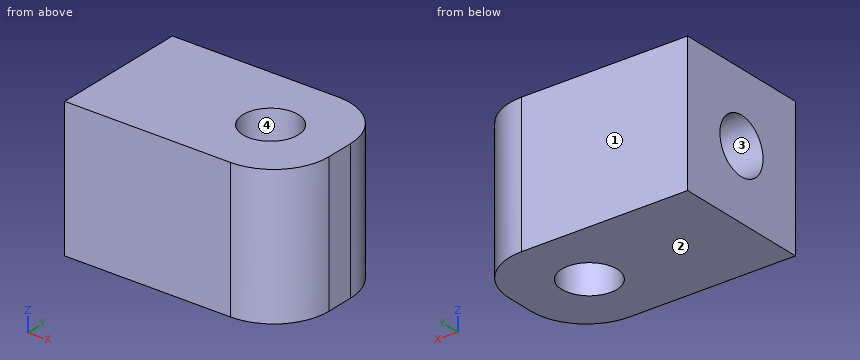
from build123d import *

# Parameters (mm, degrees)
SKETCH1_W           = 8
SKETCH1_H           = 5
BOSS_EXTRUDE1_DEPTH = 5
SKETCH2_R           = 1
CUT_EXTRUDE1_DEPTH  = 4
SKETCH3_R           = 1
CUT_EXTRUDE4_DEPTH  = 5
FILLET1_R           = 2


with BuildPart() as part:
    # Sketch1 → Boss-Extrude1 (new body)
    with BuildSketch(Plane.XY):
        with Locations((4, 2.5)):
            Rectangle(SKETCH1_W, SKETCH1_H)
    extrude(amount=BOSS_EXTRUDE1_DEPTH)

    # Sketch2 → Cut-Extrude1 (cut)
    with BuildSketch(Plane.ZY):
        with Locations((2.5, 2.5)):
            Circle(SKETCH2_R)
    extrude(amount=-CUT_EXTRUDE1_DEPTH, mode=Mode.SUBTRACT)

    # Sketch3 → Cut-Extrude4 (cut)
    with BuildSketch(Plane.XY.offset(5)):
        with Locations((5.5, 2.5)):
            Circle(SKETCH3_R)
    extrude(amount=-CUT_EXTRUDE4_DEPTH, mode=Mode.SUBTRACT)

    # Fillet1
    fillet1_edges = [part.edges().sort_by_distance(p)[0] for p in [
        (8, 5, 2.5),
        (8, 0, 2.5),
    ]]
    fillet(fillet1_edges, radius=FILLET1_R)


solid = part.part
Check sheet for the modelled part. Datum: model origin and axes. Units: mm. Face numbers are marked on the shaded views. Give positions to 0.01 mm unless a question says otherwise; leave off trailing zeros. Order: outer loops, then holes, each group sorted by start corner. A loop starts at its lowest first (then second) coordinate and runs counter-clockwise, first axis right, second up. Notation, with made-up numbers: (69.5, 21.5) - (122.5, 21.5) arc R18 ccw to (122.5, 41.5) - close; hole circle Ø1 at (-4, -19.5). An arc over 180 degrees is marked (long way). Answer as CSV lines item,"result".
1. Section check D-D (z = 3.75). Record the boundary of the cut face in (x, y).
Result sheet:
outline,"(0, 0) - (6, 0) arc R2 ccw to (8, 2) - (8, 3) arc R2 ccw to (6, 5) - (0, 5) - close; hole circle Ø2 at (5.5, 2.5)"
2. Section check A-A (x = 5.5). Record the boundary of the cut face in (y, z), then the cut area to 3 significant figures.
Result sheet:
outline,"(0, 0) - (1.5, 0) - (1.5, 5) - (0, 5) - close; (3.5, 0) - (5, 0) - (5, 5) - (3.5, 5) - close"
area,"15.0 mm²"
3. Mould release check, pull along Y, two halves, no side actions. Record for the marked faces 1, 2, 3 and 4: released by +Y, released by -Y, zero draft, split by the parting line, or undercut.
Result sheet:
face 1,"released by +Y"
face 2,"zero draft"
face 3,"undercut"
face 4,"undercut"
4. Scan lines: probe 1 along Y at (x, z) = (5.5, 2.75); probe 2 along X at (y, z) = (2.85, 2.2); probe 3 along Z at (x, y) = (3, 3.15). Record each from-to range of solid material in increasing order. Write a range as from..to.
Result sheet:
probe 1,"0..1.5, 3.5..5"
probe 2,"4..4.56, 6.44..8"
probe 3,"0..1.74, 3.26..5"
5. Section check B-B (z = 2.5). Record the boundary of the cut face in (x, y).
Result sheet:
outline,"(0, 0) - (6, 0) arc R2 ccw to (8, 2) - (8, 3) arc R2 ccw to (6, 5) - (0, 5) - (0, 3.5) - (4, 3.5) - (4, 1.5) - (0, 1.5) - close; hole circle Ø2 at (5.5, 2.5)"
6. Section check C-C (y = 2.5). Record the boundary of the cut face in (x, z), then the cut area to 3 significant figures.
Result sheet:
outline,"(0, 0) - (4.5, 0) - (4.5, 5) - (0, 5) - (0, 3.5) - (4, 3.5) - (4, 1.5) - (0, 1.5) - close; (6.5, 0) - (8, 0) - (8, 5) - (6.5, 5) - close"
area,"22.0 mm²"
